Geometry check sheet. Reference: the model listing, model coordinates, mm. A direction names the side the tool comes from. Give positions to 0.01 mm unless a question says otherwise; leave off trailing zeros. Order: outer loops, then holes, each group sorted by start corner. A loop starts at its lowest first (then second) coordinate and runs counter-clockwise, first axis right, second up.
from build123d import *

# Parameters (mm, degrees)
SKETCH_1_R          = 3
EXTRUDE_1_DEPTH     = 5
SKETCH_3_W          = 12
SKETCH_3_H          = 7
SKETCH_3_W_2        = 10
SKETCH_3_H_2        = 5
EXTRUDE_1_2_DEPTH   = 5
CUT_EXTRUDE_2_REACH = 59.51
SKETCH_4_R          = 1.2
SKETCH_5_R          = 9
CUT_EXTRUDE_3_DEPTH = 1.5
SKETCH_6_R          = 0.5
CUT_EXTRUDE_4_DEPTH = 5
SKETCH_7_R          = 2.25
CUT_EXTRUDE_5_DEPTH = 1


with BuildPart() as part:
    # 草图1 → Extrude 1 (new body)
    with BuildSketch(Plane.XY):
        with BuildLine():
            Line((-10, 5), (10, 5))
            Line((10, 5), (39.072912811, 12.790063509))
            ThreePointArc((39.072912811, 12.790063509), (55.741248097, 0), (39.072912811, -12.790063509))
            Line((39.072912811, -12.790063509), (10, -5))
            Line((10, -5), (-10, -5))
            Line((-10, -5), (-39.072912811, -12.790063509))
            ThreePointArc((-39.072912811, -12.790063509), (-55.741248097, 0), (-39.072912811, 12.790063509))
            Line((-39.072912811, 12.790063509), (-10, 5))
        make_face()
        with Locations((-42.5, 0)):
            Circle(SKETCH_1_R, mode=Mode.SUBTRACT)
        with Locations((42.5, 0)):
            Circle(SKETCH_1_R, mode=Mode.SUBTRACT)
    extrude(amount=EXTRUDE_1_DEPTH)

    # 草图3 → Extrude 1 2 (add)
    with BuildSketch(Plane(origin=(0, 0, 0), x_dir=(-1, 0, 0), z_dir=(0, 0, -1))):
        Rectangle(SKETCH_3_W, SKETCH_3_H)
        Rectangle(SKETCH_3_W_2, SKETCH_3_H_2, mode=Mode.SUBTRACT)
    extrude(amount=EXTRUDE_1_2_DEPTH)

    # 草图4 → 切除-拉伸2 (cut, up to next)
    with BuildSketch(Plane(origin=(0, 0, 0), x_dir=(-1, 0, 0), z_dir=(0, 0, -1)), mode=Mode.PRIVATE) as cut_extrude_2_sk1:
        Circle(SKETCH_4_R)
    cut_extrude_2_tool1 = extrude(cut_extrude_2_sk1.sketch, amount=-CUT_EXTRUDE_2_REACH, mode=Mode.PRIVATE) & part.part
    add(cut_extrude_2_tool1.solids().sort_by_distance((0, 0, 0))[0], mode=Mode.SUBTRACT)

    # 草图5 → 切除-拉伸3 (cut)
    with BuildSketch(Plane(origin=(0, 0, 0), x_dir=(-1, 0, 0), z_dir=(0, 0, -1))):
        with Locations((-42.5, 0)):
            Circle(SKETCH_5_R)
        with Locations((42.5, 0)):
            Circle(SKETCH_5_R)
    extrude(amount=-CUT_EXTRUDE_3_DEPTH, mode=Mode.SUBTRACT)

    # 草图6 → 切除-拉伸4 (cut)
    with BuildSketch(Plane(origin=(0, 0, 1.5), x_dir=(-1, 0, 0), z_dir=(0, 0, -1))):
        with Locations((-50, 0)):
            Circle(SKETCH_6_R)
        with Locations((-35, 0)):
            Circle(SKETCH_6_R)
        with Locations(Location((35, 0, 0), (0, 0, 180))):
            Circle(SKETCH_6_R)
        with Locations(Location((50, 0, 0), (0, 0, 180))):
            Circle(SKETCH_6_R)
    extrude(amount=-CUT_EXTRUDE_4_DEPTH, mode=Mode.SUBTRACT)

    # 草图7 → 切除-拉伸5 (cut)
    with BuildSketch(Plane.XY.offset(5)):
        with Locations((-50, 0)):
            Circle(SKETCH_7_R)
        with Locations((-35, 0)):
            Circle(SKETCH_7_R)
        with Locations((35, 0)):
            Circle(SKETCH_7_R)
        with Locations((50, 0)):
            Circle(SKETCH_7_R)
    extrude(amount=-CUT_EXTRUDE_5_DEPTH, mode=Mode.SUBTRACT)


solid = part.part
Item 1: Sectioned sample at A-A (x = 0). Enter the section's corners in (y, z), and give its area (3 significant figures).
Reported:
outline: (-5, 0) - (-3.5, 0) - (-3.5, -5) - (-2.5, -5) - (-2.5, 0) - (-1.2, 0) - (-1.2, 5) - (-5, 5) - close; (1.2, 0) - (2.5, 0) - (2.5, -5) - (3.5, -5) - (3.5, 0) - (5, 0) - (5, 5) - (1.2, 5) - close
area: 48.0 mm2
Item 2: Gauge pin test, flat ends, axial feed: pin 1 (1.5 mm diameter, centred on x = -2.5, z = 1.5, fed in from -Y); pin 2 (1.5 mm diameter, centred on x = 0.5, z = -3.5, fed in from +Y); pin 3 (1 mm diameter, centred on y = -1.5, z = 1, fed in from +X). Record the tip position at first contact, or that the pin passes through.
Reported:
pin 1: stops at y = -5
pin 2: stops at y = 3.5
pin 3: stops at x = 55.7
Item 3: Sectioned sample at C-C (x = -42.5). Enter the section's corners in (y, z).
Reported:
outline: (-13.24, 0) - (-9, 0) - (-9, 1.5) - (-3, 1.5) - (-3, 5) - (-13.24, 5) - close; (3, 1.5) - (9, 1.5) - (9, 0) - (13.24, 0) - (13.24, 5) - (3, 5) - close
Item 4: Draft check along X on faces 1 (the cylindrical face through (-0.65, 1.01, 2.46)), 2 (the flat face through (0, 3.5, -2)). Enter one of: released by +X, released by -X, zero draft, split by the parting line, or undercut.
Reported:
face 1: undercut
face 2: zero draft
Item 5: Sectioned sample at D-D (x = -18). Enter the section's corners in (y, z), and give its area (3 significant figures).
Reported:
outline: (-7.14, 0) - (7.14, 0) - (7.14, 5) - (-7.14, 5) - close
area: 71.4 mm2
Item 6: Set-up check for faces 3 (the flat face through (0, -3.5, -2)), 4 (the flat face through (5, 0, -2)), 5 (the flat face through (0, 5, 2)), 6 (the cylindrical face through (47.752, 0.099, 4.507)), 7 (the flat face through (0, -5, 2)): record each of +Z, -Z, +X, -X, +Y, -Y from which the full face is reachable in a straight line by a thin tool's end or side.
Reported:
face 3: -Z, +X, -X, -Y
face 4: -Z
face 5: +Z, -Z, +Y
face 6: +Z
face 7: +Z, -Z, -Y
Item 7: Sectioned sample at B-B (y = 7). Enter the section's corners in (x, z).
Reported:
outline: (-53.74, 0) - (-48.16, 0) - (-48.16, 1.5) - (-36.84, 1.5) - (-36.84, 0) - (-17.46, 0) - (-17.46, 5) - (-53.74, 5) - close; (17.46, 0) - (36.84, 0) - (36.84, 1.5) - (48.16, 1.5) - (48.16, 0) - (53.74, 0) - (53.74, 5) - (17.46, 5) - close
Item 8: Scan lines: L1, parallel to Y at x = -42.5, z = 0.5; L2, parallel to X at y = -0.5, z = 1.25; L3, parallel to Y at x = 42.5, z = 4.05. Record each from-to range of solid material in increasing order.
Reported:
L1: y = -13.24 to -9, 9 to 13.24
L2: x = -55.73 to -51.49, -33.51 to -1.09, 1.09 to 33.51, 51.49 to 55.73
L3: y = -13.24 to -3, 3 to 13.24
